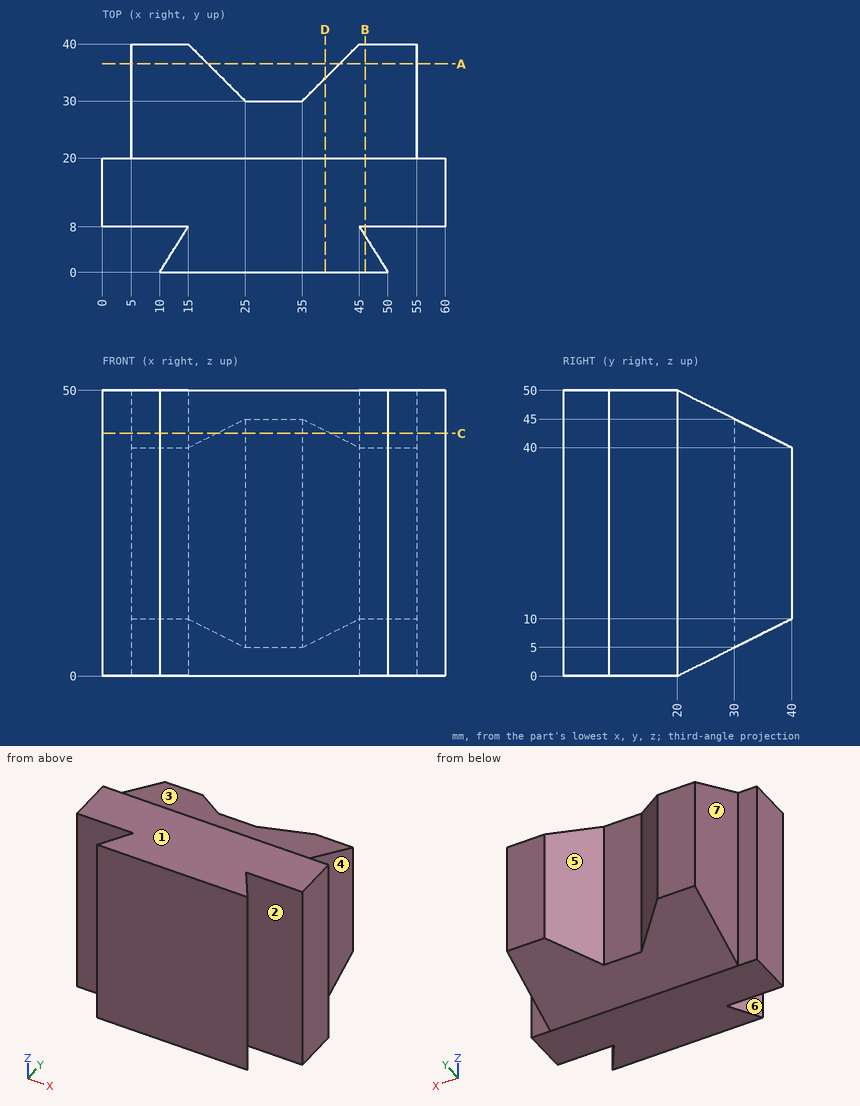
Input: dimensioned drawing with shaded views. Units: mm. Origin: part minimum x, y, z. A direction names the side the tool comes from. Coordinates: 2 decimals unless noted, no trailing zeros. Loops run counter-clockwise (first coordinate to the right, second up) from the corner with the lowest first, then second, coordinate; pieces in that order, holes last. Notation, with made-up numbers: (76.25, 38) -> (87.25, 38) arc R19 ccw to (87.25, 74) -> close; hole circle Ø5 at (-10, -34). An arc over 180 degrees is marked (long way). One line per item, written item: value. Start each with the question number.
Q1. Line query: line 1 along X through (y, z) = (35, 35.5); line 2 along X through (y, z) = (27, 19); line 3 along Y through (x, z) = (8, 7.5). Output: solid intervals per line, ascending.
Q2. Section query D-D, the plane x = 39. Return the cut outline in (y, z).
Q3. Section query B-B, the plane x = 46. Return the cut outline in (y, z).
Q4. Section query A-A, the plane y = 36.5. Return the cut outline in (x, z).
Q5. Contact query for flat-ended pins moving along their axis: P1, Ø10, axis at y = 34.5, z = 20.5, coming from the +X side; P2, Ø11, axis at x = 30.5, z = 16, coming from the +Y side; P3, Ø10, axis at y = 32.5, z = 35.5, coming from the -X side. Output: stop coordinate, or through.
Q6. Set-up query: the marked faces 4, 5, 6 and 7. Return all of +Z, -Z, +X, -X, +Y, -Y with unobstructed straight access to the full face (end or side cutting, diameter ignored); none if empty.
Q7. Mould query, pull axis Y, two halves, no side actions, for the marked faces 1, 2 and 3. Classes: pulls with the +Y half, pulls with the -Y half, needs draft (parallel to the pull), parting line crosses it, or undercut.
Q8. Section query C-C, the plane z = 42.5. Return the cut outline in (x, y).
Results:
1. line 1: 5 to 20, 40 to 55
1. line 2: 5 to 55
1. line 3: 8 to 35
2. outline: (0, 0) -> (20, 0) -> (34, 7) -> (34, 43) -> (20, 50) -> (0, 50) -> close
3. outline: (0, 0) -> (6.4, 0) -> (6.4, 50) -> (0, 50) -> close; (8, 0) -> (20, 0) -> (40, 10) -> (40, 40) -> (20, 50) -> (8, 50) -> close
4. outline: (5, 8.25) -> (18.5, 8.25) -> (18.5, 41.75) -> (5, 41.75) -> close; (41.5, 8.25) -> (55, 8.25) -> (55, 41.75) -> (41.5, 41.75) -> close
5. P1: x = 55
5. P2: y = 31
5. P3: x = 5
6. face 4: +Z, -Z, +X, +Y
6. face 5: +Z, -Z, +Y
6. face 6: +Z, -Z, -X
6. face 7: +Z, -Z, -X, +Y
7. face 1: needs draft
7. face 2: undercut
7. face 3: pulls with the +Y half
8. outline: (0, 8) -> (15, 8) -> (10, 0) -> (50, 0) -> (45, 8) -> (60, 8) -> (60, 20) -> (55, 20) -> (55, 35) -> (40, 35) -> (35, 30) -> (25, 30) -> (20, 35) -> (5, 35) -> (5, 20) -> (0, 20) -> close
